The drawing under review shows one solid part. Ordinate dimensions are in mm from its lowest x, y, z. Give positions to 0.01 mm unless a question says otherwise; leave off trailing zeros. Write each loop counter-clockwise with the first axis right and the second up, starting at its lowest first coordinate (ties: lowest second). Pieces come first, ordered by that corner, then holes.
Q1. For line 1 (X direction, y = 0.3, z = 19) (1 decimal); line 2 (X direction, y = 2.75, z = 20); line 3 (Z direction, x = 22.5, y = 0.35), list the stretches that pass through material, from the lowest coordinate up.
Q2. Mouldability with a two-part tool opening along X and no side actions: class the marked faces 1, 2, 3 and 4 as released by +X, released by -X, zero draft, split by the parting line, or undercut.
Q3. We need section C-C (y = 0.9). Write out the cut boundary in (x, z).
Q4. We need section A-A (z = 20). Give the number of separate pieces and of enclosed holes in the cut face.
Q5. Insertion check: P1, Ø17.5, axis at x = 20, z = 20, coming from the +Y side; P2, Ø1.5, axis at y = 3.5, z = 12.5, coming from the +X side; P3, Ø3, axis at x = 24.5, y = 4, coming from the -Z side; P4, Ø1.5, axis at y = 2, z = 34.5, coming from the -X side. Each pin has a flat end and moves straight along its axis. Give the tip position at first contact, or say it passes through.
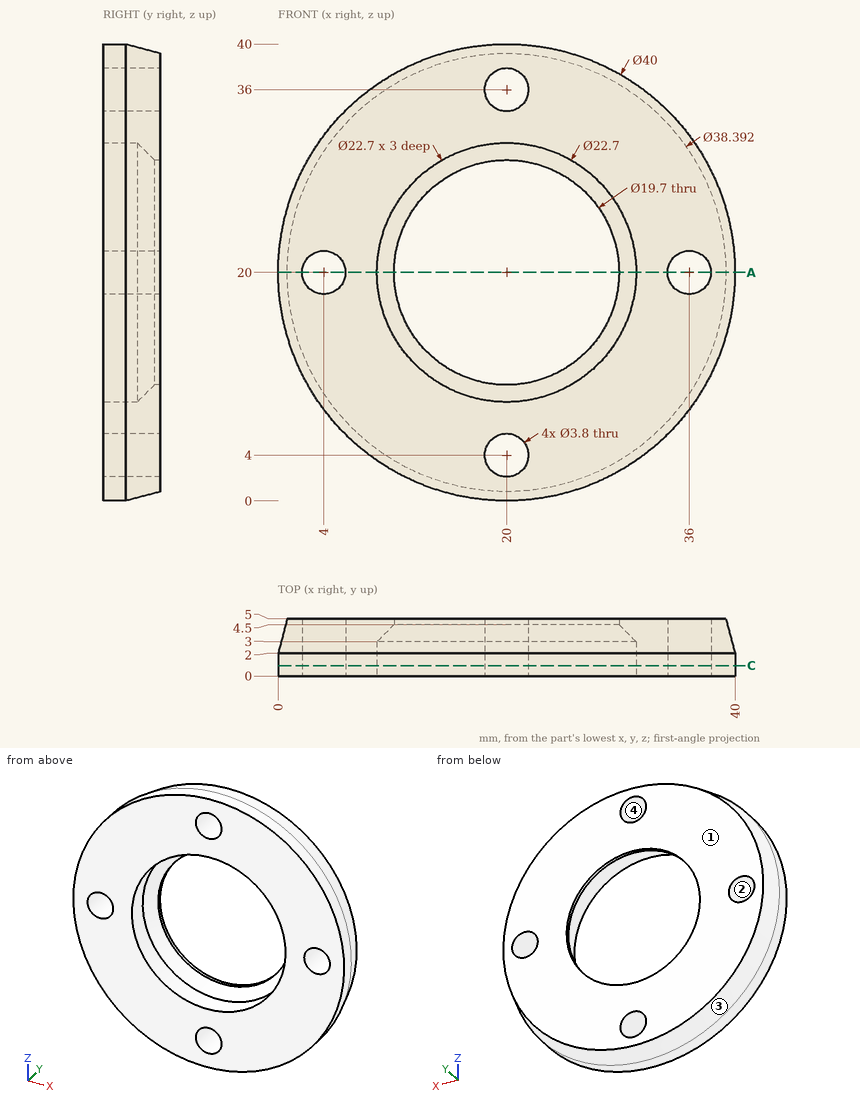
Computed:
1. line 1: x = 0 to 2.4, 5.6 to 8.7, 31.3 to 34.4, 37.6 to 40
1. line 2: x = 0.2 to 2.1, 5.9 to 8.65, 31.35 to 34.1, 37.9 to 39.8
1. line 3: z = 0.16 to 8.93, 31.07 to 39.84
2. face 1: zero draft
2. face 2: undercut
2. face 3: split by the parting line
2. face 4: undercut
3. outline: circle Ø40 at (20, 20); hole circle Ø3.8 at (4, 20); hole circle Ø22.7 at (20, 20); hole circle Ø3.8 at (20, 4); hole circle Ø3.8 at (20, 36); hole circle Ø3.8 at (36, 20)
4. separate pieces: 4
4. enclosed holes: 0
5. P1: passes through
5. P2: stops at x = 38.47
5. P3: stops at z = 0.54
5. P4: stops at x = 5.48
